The model under review builds one solid part; all positions refer to its coordinate system, in mm. A direction names the side the tool comes from. Coordinates: 2 decimals unless noted, no trailing zeros. Loops run counter-clockwise (first coordinate to the right, second up) from the corner with the lowest first, then second, coordinate; pieces in that order, holes last. Notation, with made-up numbers: M 77,53.5 L 123,53.5 A10 cw 123,63.5 Z; hole C 19.5,0 d11. An arc over 180 degrees is marked long. Use one line per item in the form item = value.
```python
from build123d import *

# Parameters (mm, degrees)
BOSS_EXTRUDE2_DEPTH = 2
BOSS_EXTRUDE3_DEPTH = 10
CUT_EXTRUDE1_REACH  = 31.394
CUT_EXTRUDE2_REACH  = 21.698
SKETCH5_R           = 4.15
SKETCH6_W           = 20
SKETCH6_H           = 3.6
CUT_EXTRUDE3_DEPTH  = 1
FILLET1_R           = 1
CUT_EXTRUDE4_START  = -0.8
CUT_EXTRUDE4_DEPTH  = 0.8
SKETCH8_W           = 13.4
SKETCH8_H           = 1.173218526
BOSS_EXTRUDE4_DEPTH = 1.3
SKETCH10_W          = 0.69
SKETCH10_H          = 1.173218526
BOSS_EXTRUDE5_DEPTH = 2
FILLET2_R           = 0.5
FILLET6_R           = 0.5
FILLET8_R           = 1.5
CUT_EXTRUDE6_DEPTH  = 22.5
FILLET9_R           = 0.2


with BuildPart() as part:
    # Sketch2 → Boss-Extrude2 (new body)
    with BuildSketch(Plane(origin=(0, 0, 0), x_dir=(1, 0, 0), z_dir=(0, 1, 0))):
        with BuildLine():
            Line((-10, -12), (10, -12))
            ThreePointArc((10, -12), (11.414213562, -11.414213562), (12, -10))
            Line((12, -10), (12, 10))
            ThreePointArc((12, 10), (11.414213562, 11.414213562), (10, 12))
            Line((10, 12), (-10, 12))
            ThreePointArc((-10, 12), (-11.414213562, 11.414213562), (-12, 10))
            Line((-12, 10), (-12, -10))
            ThreePointArc((-12, -10), (-11.414213562, -11.414213562), (-10, -12))
        make_face()
    extrude(amount=BOSS_EXTRUDE2_DEPTH)

    # Sketch3 → Boss-Extrude3 (add)
    with BuildSketch(Plane(origin=(0, 2, 0), x_dir=(1, 0, 0), z_dir=(0, 1, 0))):
        with BuildLine():
            Line((-10, -12), (10, -12))
            ThreePointArc((10, -12), (11.414213562, -11.414213562), (12, -10))
            Line((12, -10), (12, 10))
            ThreePointArc((12, 10), (11.414213562, 11.414213562), (10, 12))
            Line((10, 12), (-10, 12))
            ThreePointArc((-10, 12), (-11.414213562, 11.414213562), (-12, 10))
            Line((-12, 10), (-12, -10))
            ThreePointArc((-12, -10), (-11.414213562, -11.414213562), (-10, -12))
        make_face()
        with BuildLine():
            Line((-9.5, -10), (9.5, -10))
            ThreePointArc((9.5, -10), (9.853553391, -9.853553391), (10, -9.5))
            Line((10, -9.5), (10, 9.5))
            ThreePointArc((10, 9.5), (9.853553391, 9.853553391), (9.5, 10))
            Line((9.5, 10), (-9.5, 10))
            ThreePointArc((-9.5, 10), (-9.853553391, 9.853553391), (-10, 9.5))
            Line((-10, 9.5), (-10, -9.5))
            ThreePointArc((-10, -9.5), (-9.853553391, -9.853553391), (-9.5, -10))
        make_face(mode=Mode.SUBTRACT)
    extrude(amount=BOSS_EXTRUDE3_DEPTH)

    # Sketch4 → Cut-Extrude1 (cut, up to next)
    with BuildSketch(Plane.XY.offset(12), mode=Mode.PRIVATE) as cut_extrude1_sk1:
        with BuildLine():
            Line((-4.05, 7.7), (4.05, 7.7))
            ThreePointArc((4.05, 7.7), (4.403553391, 7.553553391), (4.55, 7.2))
            Line((4.55, 7.2), (4.55, 4.8))
            ThreePointArc((4.55, 4.8), (4.403553391, 4.446446609), (4.05, 4.3))
            Line((4.05, 4.3), (-4.05, 4.3))
            ThreePointArc((-4.05, 4.3), (-4.403553391, 4.446446609), (-4.55, 4.8))
            Line((-4.55, 4.8), (-4.55, 7.2))
            ThreePointArc((-4.55, 7.2), (-4.403553391, 7.553553391), (-4.05, 7.7))
        make_face()
    cut_extrude1_tool1 = extrude(cut_extrude1_sk1.sketch, amount=-CUT_EXTRUDE1_REACH, mode=Mode.PRIVATE) & part.part
    add(cut_extrude1_tool1.solids().sort_by_distance((0, 6, 12))[0], mode=Mode.SUBTRACT)

    # Sketch5 → Cut-Extrude2 (cut, up to next)
    with BuildSketch(Plane(origin=(0, 2, 0), x_dir=(1, 0, 0), z_dir=(0, 1, 0)), mode=Mode.PRIVATE) as cut_extrude2_sk1:
        with Locations(Location((0, 0, 0), (0, 0, 270))):
            Circle(SKETCH5_R)
    cut_extrude2_tool1 = extrude(cut_extrude2_sk1.sketch, amount=-CUT_EXTRUDE2_REACH, mode=Mode.PRIVATE) & part.part
    add(cut_extrude2_tool1.solids().sort_by_distance((0, 2, 0))[0], mode=Mode.SUBTRACT)

    # Sketch6 → Cut-Extrude3 (cut)
    with BuildSketch(Plane(origin=(0, 2, 0), x_dir=(1, 0, 0), z_dir=(0, 1, 0))):
        with Locations((-0.054263112, 0)):
            Rectangle(SKETCH6_W, SKETCH6_H)
    extrude(amount=-CUT_EXTRUDE3_DEPTH, mode=Mode.SUBTRACT)

    # Fillet1
    fillet1_edges = [part.edges().sort_by_distance(p)[0] for p in [
        (9.945736888, 1, 0),
        (-10.054263112, 1, 0),
    ]]
    fillet(fillet1_edges, radius=FILLET1_R - 0.0001)  # a hair under: the kernel refuses the full size

    # Sketch7 → Cut-Extrude4 (cut)
    with BuildSketch(Plane(origin=(0, 0, 10), x_dir=(-1, 0, 0), z_dir=(0, 0, -1)).offset(CUT_EXTRUDE4_START)):
        with BuildLine():
            Line((-6.05, 8.26), (-6.05, 4.3))
            Line((-6.05, 4.3), (-4.05, 4.3))
            ThreePointArc((-4.05, 4.3), (-4.403553391, 4.446446609), (-4.55, 4.8))
            Line((-4.55, 4.8), (-4.55, 7.2))
            ThreePointArc((-4.55, 7.2), (-4.403553391, 7.553553391), (-4.05, 7.7))
            Line((-4.05, 7.7), (4.05, 7.7))
            ThreePointArc((4.05, 7.7), (4.403553391, 7.553553391), (4.55, 7.2))
            Line((4.55, 7.2), (4.55, 4.8))
            ThreePointArc((4.55, 4.8), (4.403553391, 4.446446609), (4.05, 4.3))
            Line((4.05, 4.3), (6.05, 4.3))
            Line((6.05, 4.3), (6.05, 8.26))
            Line((6.05, 8.26), (-6.05, 8.26))
        make_face()
        Polygon((-6.05, 4.3), (-6.05, 3.3), (6.05, 3.3), (6.05, 4.3), (4.05, 4.3), (-4.05, 4.3), align=None)
    extrude(amount=CUT_EXTRUDE4_DEPTH, mode=Mode.SUBTRACT)

    # Sketch8 → Boss-Extrude4 (add)
    with BuildSketch(Plane(origin=(0, 2, 0), x_dir=(1, 0, 0), z_dir=(0, 1, 0))):
        with Locations((0, -4.736609263)):
            Rectangle(SKETCH8_W, SKETCH8_H)
    extrude(amount=BOSS_EXTRUDE4_DEPTH)

    # Sketch10 → Boss-Extrude5 (add)
    with BuildSketch(Plane(origin=(0, 3.3, 0), x_dir=(1, 0, 0), z_dir=(0, 1, 0))):
        with Locations((6.355, -4.736609263)):
            Rectangle(SKETCH10_W, SKETCH10_H)
        with Locations((-6.355, -4.736609263)):
            Rectangle(SKETCH10_W, SKETCH10_H)
    extrude(amount=BOSS_EXTRUDE5_DEPTH)

    # Fillet2
    fillet2_edges = [part.edges().sort_by_distance(p)[0] for p in [
        (-6.01, 3.3, 4.736609263),
        (6.01, 3.3, 4.736609263),
    ]]
    fillet(fillet2_edges, radius=FILLET2_R)

    # Fillet6
    fillet6_edges = [part.edges().sort_by_distance(p)[0] for p in [
        (6.7, 2, 4.736609263),
        (-6.7, 2, 4.736609263),
    ]]
    fillet(fillet6_edges, radius=FILLET6_R)

    # Fillet8
    fillet8_edges = [part.edges().sort_by_distance(p)[0] for p in [
        (-12, 12, 0),
        (-11.414213562, 12, 11.414213562),
        (11.414213562, 12, -11.414213562),
        (0, 12, -12),
        (-11.414213562, 12, -11.414213562),
        (0, 12, 12),
        (11.414213562, 12, 11.414213562),
        (12, 12, 0),
    ]]
    fillet(fillet8_edges, radius=FILLET8_R)

    # Sketch21 → Cut-Extrude6 (cut)
    with BuildSketch(Plane(origin=(0, 0, -12), x_dir=(-1, 0, 0), z_dir=(0, 0, -1))):
        with BuildLine():
            Line((-10.3, 10.26661549), (10.3, 10.26661549))
            ThreePointArc((10.3, 10.26661549), (10.441421356, 10.208036847), (10.5, 10.06661549))
            Line((10.5, 10.06661549), (10.5, 8.96661549))
            ThreePointArc((10.5, 8.96661549), (10.441421356, 8.825194134), (10.3, 8.76661549))
            Line((10.3, 8.76661549), (-10.3, 8.76661549))
            ThreePointArc((-10.3, 8.76661549), (-10.441421356, 8.825194134), (-10.5, 8.96661549))
            Line((-10.5, 8.96661549), (-10.5, 10.06661549))
            ThreePointArc((-10.5, 10.06661549), (-10.441421356, 10.208036847), (-10.3, 10.26661549))
        make_face()
    extrude(amount=-CUT_EXTRUDE6_DEPTH, mode=Mode.SUBTRACT)

    # Fillet9
    fillet9_edges = [part.edges().sort_by_distance(p)[0] for p in [
        (10.441421356, 8.825194134, 10.5),
        (10.5, 9.51661549, 10.5),
        (10.441421356, 10.208036847, 10.5),
        (-10.441421356, 8.825194134, 10.5),
        (-10.441421356, 10.208036847, 10.5),
        (-10.5, 9.51661549, 10.5),
        (0, 8.76661549, 10.5),
        (0, 10.26661549, 10.5),
    ]]
    fillet(fillet9_edges, radius=FILLET9_R)


solid = part.part
```
1. Add section D-D (z = -8). State the section outline as (x, y) points.
Response values:
outline = M -12,0 L 12,0 L 12,10.5 A1.5 ccw 10.5,12 L 10,12 L 10,10.27 L 10.3,10.27 A0.2 cw 10.5,10.07 L 10.5,8.97 A0.2 cw 10.3,8.77 L 10,8.77 L 10,2 L -10,2 L -10,8.77 L -10.3,8.77 A0.2 cw -10.5,8.97 L -10.5,10.07 A0.2 cw -10.3,10.27 L -10,10.27 L -10,12 L -10.5,12 A1.5 ccw -12,10.5 Z
2. Machinability: for faces 4 (the face through (0, 10.267, -11)), 5 (the face through (-6, 1, 0)), 6 (the face through (6.05, 5.8, 10.4)), 7 (the face through (-4.55, 6, 11)), 8 (the face through (-1.589, 1.014, 3.834)), which of the approach directions +Z, -Z, +X, -X, +Y, -Y give a long, thin tool a straight path to every point of the face, cutting with its end or side? Answer none if there is none.
Response values:
face_4 = -Z
face_5 = +Y
face_6 = none
face_7 = +Z
face_8 = +Y, -Y
3. The part is to be moulded in two halves that separate along X. For faces 1 (the face through (-10.2, 12, 0)), 2 (the face through (-11.4, 5.18, -11.43)), 3 (the face through (0, 8.767, -11)), say which applies: pulls with the +X half, pulls with the -X half, needs draft (parallel to the pull), parting line crosses it, or undercut.
Response values:
face_1 = needs draft
face_2 = pulls with the -X half
face_3 = undercut
4. Add section B-B (x = 8.25). State the section outline as (y, z) points, then the cut area to 3 significant figures.
Response values:
outline = M 0,-12 L 8.77,-12 L 8.77,-10 L 2,-10 L 2,-1.8 L 1,-1.8 L 1,1.8 L 2,1.8 L 2,10 L 8.77,10 L 8.77,10.3 A0.2 cw 8.97,10.5 L 10.07,10.5 A0.2 cw 10.27,10.3 L 10.27,10 L 12,10 L 12,10.5 A1.5 ccw 10.5,12 L 0,12 Z; M 10.27,-12 L 10.5,-12 A1.5 ccw 12,-10.5 L 12,-10 L 10.27,-10 Z
area = 79.7 mm^2
5. Wall thickness on line 1 along Z through (x, y) = (0, 1.2); line 2 along X through (y, z) = (2.5, -8): over which ranges is each line inside the solid? List them lowest first. Write a range as from..to.
Response values:
line_1 = -12..-4.15, 4.15..12
line_2 = -12..-10, 10..12
6. Add section C-C (y = 1.5). State the section outline as (x, z) points, then the cut area to 3 significant figures.
Response values:
outline = M -12,-10 A2 ccw -10,-12 L 10,-12 A2 ccw 12,-10 L 12,10 A2 ccw 10,12 L -10,12 A2 ccw -12,10 Z; hole M -9.92,-1.8 L -3.74,-1.8 A4.15 ccw 3.74,-1.8 L 9.81,-1.8 L 9.81,1.8 L 3.74,1.8 A4.15 ccw -3.74,1.8 L -9.92,1.8 Z
area = 476 mm^2
7. Insertion check: P1, Ø0.6, axis at y = 6, z = 11.5, coming from the -X side; P2, Ø0.5, axis at y = 11, z = 0, coming from the +X side. Each pin has a flat end and moves straight along its axis. Give the tip position at first contact, or say it passes through.
Response values:
P1 = -11.6
P2 = 11.98
